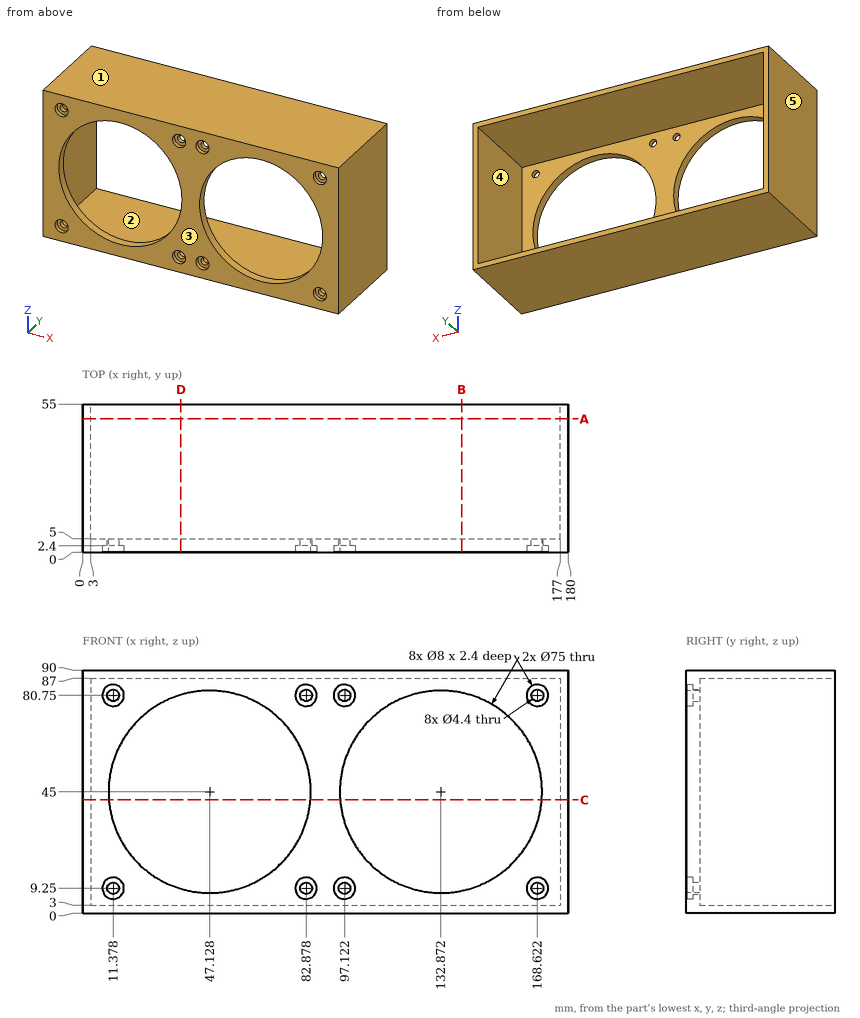
Design review of the part shown in the three views and the two pictorial views. Dimensions are in mm from the part's minimum x, y and z. A direction names the side the tool comes from. Round coordinates to 2 decimals unless told otherwise and drop trailing zeros. Loops run counter-clockwise (first coordinate to the right, second up) from the corner with the lowest first, then second, coordinate; pieces in that order, holes last.
Q1. Insertion check: pin 1 Ø5 at (x, z) = (90, 46.5) entering from +Y; pin 2 Ø4 at (x, z) = (82.88, 80.75) entering from +Y; pin 3 Ø5 at (x, z) = (82.88, 80.75) entering from -Y. Each pin has a flat end and moves straight along its axis. Give the tip position at first contact, or say it passes through.
Result sheet:
pin 1: stops at y = 5
pin 2: passes through
pin 3: stops at y = 2.4
Q2. To check wall thickness, follow line 1 along Z through (x, y) = (77, 21.5); line 2 along X through (y, z) = (8.5, 16); line 3 along X through (y, z) = (3, 43). State the ranges of each line that lie inside material, in increasing order.
Result sheet:
line 1: z = 0 to 3, 87 to 90
line 2: x = 0 to 3, 177 to 180
line 3: x = 0 to 9.68, 84.57 to 95.43, 170.32 to 180
Q3. Machinability: for the marked faces 1 and 2, which of the approach directions +Z, -Z, +X, -X, +Y, -Y give a long, thin tool a straight path to every point of the face, cutting with its end or side? Answer none if there is none.
Result sheet:
face 1: +Z, +X, -X, +Y, -Y
face 2: +Y
Q4. Mouldability with a two-part tool opening along X and no side actions: class the marked faces 3, 4 and 5 as +X half, -X half, draft (parallel to the pull), parting line (faces both ways), or undercut.
Result sheet:
face 3: draft
face 4: undercut
face 5: -X half
Q5. Add section B-B on x = 140.5. Write out the cut boundary in (y, z), plus the area to 3 significant figures.
Result sheet:
outline: (0, 0) - (55, 0) - (55, 3) - (5, 3) - (5, 8.28) - (0, 8.28) - close; (0, 81.72) - (5, 81.72) - (5, 87) - (55, 87) - (55, 90) - (0, 90) - close
area: 383 mm2
Q6. Add section C-C on z = 42. Write out the cut boundary in (x, y).
Result sheet:
outline: (0, 0) - (9.75, 0) - (9.75, 5) - (3, 5) - (3, 55) - (0, 55) - close; (84.51, 0) - (95.49, 0) - (95.49, 5) - (84.51, 5) - close; (170.25, 0) - (180, 0) - (180, 55) - (177, 55) - (177, 5) - (170.25, 5) - close
Q7. Add section D-D on x = 36.5. Write out the cut boundary in (y, z).
Result sheet:
outline: (0, 0) - (55, 0) - (55, 3) - (5, 3) - (5, 9.04) - (0, 9.04) - close; (0, 80.96) - (5, 80.96) - (5, 87) - (55, 87) - (55, 90) - (0, 90) - close
Q8. Add section A-A on y = 49.5. Write out the cut boundary in (x, z), plus the area to 3 significant figures.
Result sheet:
outline: (0, 0) - (180, 0) - (180, 90) - (0, 90) - close; hole (3, 3) - (177, 3) - (177, 87) - (3, 87) - close
area: 1,580 mm2
